Check sheet for the modelled part. Datum: model origin and axes. Units: mm. Coordinates: 2 decimals unless noted, no trailing zeros. Loops run counter-clockwise (first coordinate to the right, second up) from the corner with the lowest first, then second, coordinate; pieces in that order, holes last. Notation, with made-up numbers: (-12, 10.5) -> (37, 10.5) arc R25 ccw to (37, 26.5) -> close; hole circle Ø8 at (-23.5, 53.25). An arc over 180 degrees is marked (long way). Use CSV: the item, a comma, the result in double quotes. Start each with the question number.
1. Thickness scan on L1, parallel to X at y = 5.25, z = -17.5; L2, parallel to X at y = 5.5, z = 17.5; L3, parallel to X at y = 2.75, z = 12. Record the ranges inside material, lowest first.
2. Sectioned sample at B-B, the plane z = -17.5. Record the cut outline in (x, y), and give its area (3 significant figures).
3. Gauge pin test, flat end, axial feed: pin 1 (1.2 mm diameter, centred on x = -12, z = -18, fed in from -Y). Record the tip position at first contact, or that the pin passes through.
4. Sectioned sample at A-A, the plane x = 12. Record the cut outline in (y, z).
```python
from build123d import *

# Parameters (mm, degrees)
BOSS_EXTRUDE1_DEPTH = 23
SKETCH2_R           = 2
CUT_EXTRUDE1_DEPTH  = 7.5


with BuildPart() as part:
    # Sketch1 → Boss-Extrude1 (new, symmetric)
    with BuildSketch(Plane.XY):
        with BuildLine():
            Line((-27, 0), (27, 0))
            ThreePointArc((27, 0), (29.121320344, 0.878679656), (30, 3))
            Line((30, 3), (30, 7))
            ThreePointArc((30, 7), (29.121320344, 9.121320344), (27, 10))
            Line((27, 10), (-27, 10))
            ThreePointArc((-27, 10), (-29.121320344, 9.121320344), (-30, 7))
            Line((-30, 7), (-30, 3))
            ThreePointArc((-30, 3), (-29.121320344, 0.878679656), (-27, 0))
        make_face()
    extrude(amount=BOSS_EXTRUDE1_DEPTH, both=True)

    # Sketch2 → Cut-Extrude1 (cut)
    with BuildSketch(Plane(origin=(0, 0, 0), x_dir=(1, 0, 0), z_dir=(0, 1, 0))):
        with Locations(Location((12, -17.5, 0), (0, 0, 270))):
            Circle(SKETCH2_R)
        with Locations(Location((-12, 17.5, 0), (0, 0, 270))):
            Circle(SKETCH2_R)
    extrude(amount=CUT_EXTRUDE1_DEPTH, mode=Mode.SUBTRACT)


solid = part.part
```
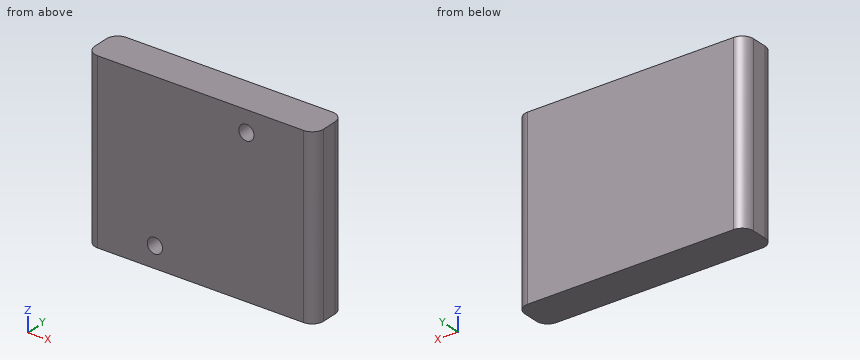
Completed:
1,L1,"-30 to -14, -10 to 30"
1,L2,"-30 to 10, 14 to 30"
1,L3,"-29.99 to 29.99"
2,outline,"(-30, 3) arc R3 ccw to (-27, 0) -> (-14, 0) -> (-14, 7.5) -> (-10, 7.5) -> (-10, 0) -> (27, 0) arc R3 ccw to (30, 3) -> (30, 7) arc R3 ccw to (27, 10) -> (-27, 10) arc R3 ccw to (-30, 7) -> close"
2,area,"562 mm²"
3,pin 1,"y = 7.5"
4,outline,"(0, -23) -> (10, -23) -> (10, 23) -> (0, 23) -> (0, 19.5) -> (7.5, 19.5) -> (7.5, 15.5) -> (0, 15.5) -> close"
